from build123d import *

# Parameters (mm, degrees)
CROQUIS1_W                 = 48.280426218
CROQUIS1_H                 = 21.608022922
SALIENTE_EXTRUIR1_DEPTH    = 5
CROQUIS2_R                 = 2.974152903
CORTAR_EXTRUIR1_DEPTH      = 15
CORTAR_EXTRUIR1_DEPTH_BACK = 23
CROQUIS3_R                 = 3.556
CORTAR_EXTRUIR2_DEPTH      = 31.496
CORTAR_EXTRUIR2_DEPTH_BACK = 20.828
CROQUIS4_R                 = 3.556
CORTAR_EXTRUIR3_DEPTH      = 8.636
CORTAR_EXTRUIR3_DEPTH_BACK = 20.828
CROQUIS5_R                 = 4.117290135
SALIENTE_EXTRUIR2_DEPTH    = 8.636


with BuildPart() as part:
    # Croquis1 → Saliente-Extruir1 (new body)
    with BuildSketch(Plane(origin=(0, 0, 0), x_dir=(1, 0, 0), z_dir=(0, 1, 0))):
        Rectangle(CROQUIS1_W, CROQUIS1_H)
    extrude(amount=SALIENTE_EXTRUIR1_DEPTH)

    # Croquis2 → Cortar-Extruir1 (cut, two sides)
    with BuildSketch(Plane(origin=(0, 0, 0), x_dir=(1, 0, 0), z_dir=(0, 1, 0))) as cortar_extruir1_sk:
        with Locations((18.312839715, 0)):
            Circle(CROQUIS2_R)
        with Locations((-18.312839715, 0)):
            Circle(CROQUIS2_R)
    extrude(amount=CORTAR_EXTRUIR1_DEPTH, mode=Mode.SUBTRACT)
    extrude(cortar_extruir1_sk.sketch, amount=-CORTAR_EXTRUIR1_DEPTH_BACK, mode=Mode.SUBTRACT)

    # Croquis3 → Cortar-Extruir2 (cut, two sides)
    with BuildSketch(Plane(origin=(0, 0, 0), x_dir=(1, 0, 0), z_dir=(0, 1, 0))) as cortar_extruir2_sk:
        with Locations((18.312839715, 0)):
            Circle(CROQUIS3_R)
    extrude(amount=CORTAR_EXTRUIR2_DEPTH, mode=Mode.SUBTRACT)
    extrude(cortar_extruir2_sk.sketch, amount=-CORTAR_EXTRUIR2_DEPTH_BACK, mode=Mode.SUBTRACT)

    # Croquis4 → Cortar-Extruir3 (cut, two sides)
    with BuildSketch(Plane(origin=(0, 5, 0), x_dir=(1, 0, 0), z_dir=(0, 1, 0))) as cortar_extruir3_sk:
        with Locations((-18.312839715, 0)):
            Circle(CROQUIS4_R)
    extrude(amount=CORTAR_EXTRUIR3_DEPTH, mode=Mode.SUBTRACT)
    extrude(cortar_extruir3_sk.sketch, amount=-CORTAR_EXTRUIR3_DEPTH_BACK, mode=Mode.SUBTRACT)

    # Croquis5 → Saliente-Extruir2 (add)
    with BuildSketch(Plane.XY):
        Polygon((7.112251642, 9.190063188), (3.556125821, 15.349453788), (-3.556125821, 15.349453788), (-7.112251642, 9.190063188), (-3.556125821, 3.030672588), (3.556125821, 3.030672588), align=None)
        with Locations((0, 9.190063188)):
            Circle(CROQUIS5_R, mode=Mode.SUBTRACT)
    extrude(amount=SALIENTE_EXTRUIR2_DEPTH)


solid = part.part
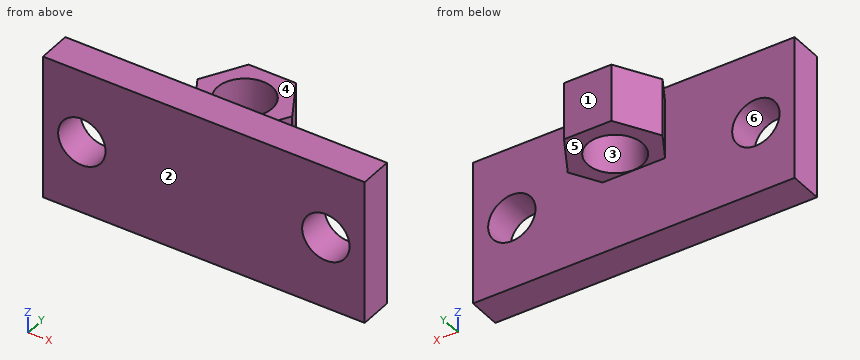
Model file for the job. Use its own axes, mm. Face numbers are marked on the shaded views. A direction names the side the tool comes from. Give positions to 0.01 mm unless a question says otherwise; leave off trailing zeros. Order: outer loops, then holes, each group sorted by start corner. A loop starts at its lowest first (then second) coordinate and runs counter-clockwise, first axis right, second up. Notation, with made-up numbers: (6, 54) - (41, 54) arc R10 cw to (41, 62) - close; hole circle Ø4 at (36.5, 12). An arc over 180 degrees is marked (long way). Return JSON: item names as keys, results as strings.
1) Flat gauge pins, fed straight in: P1, Ø8, axis at x = -0.5, y = 10, coming from the +Z side; P2, Ø3, axis at x = 1.5, z = 0.5, coming from the -Y side; P3, Ø11.5, axis at x = 18.31, z = 0, coming from the +Y side; P4, Ø5, axis at x = 9.5, y = 8, coming from the +Z side. Where does each tip first touch, or does it go through?
Geometry says:
{"P1": "z = 8.64", "P2": "y = 0", "P3": "y = 5", "P4": "through"}
2) Cut at B-B, the plane z = 3. Give the cut face in (x, y), plus the area to 3 significant figures.
Geometry says:
{"outline": "(-24.14, 0) - (-20.22, 0) - (-20.22, 5) - (-24.14, 5) - close; (-16.4, 0) - (16.4, 0) - (16.4, 5) - (4.69, 5) - (7.11, 9.19) - (3.56, 15.35) - (-3.56, 15.35) - (-7.11, 9.19) - (-4.69, 5) - (-16.4, 5) - close; (20.22, 0) - (24.14, 0) - (24.14, 5) - (20.22, 5) - close; hole circle Ø8.23 at (0, 9.19)", "area": "265 mm²"}
3) Cut at A-A, the plane x = 0. Give the cut face in (y, z), plus the area to 3 significant figures.
Geometry says:
{"outline": "(0, -10.8) - (5, -10.8) - (5, 0) - (5.07, 0) - (5.07, 8.64) - (5, 8.64) - (5, 10.8) - (0, 10.8) - close; (13.31, 0) - (15.35, 0) - (15.35, 8.64) - (13.31, 8.64) - close", "area": "126 mm²"}
4) Probe line 1 (X direction, y = 3.75, z = 0); line 2 (Y direction, x = 12, z = 0.75); line 3 (Y direction, x = 0, z = 3.5). List the from-to ranges inside material, lowest first. Write a range as from..to.
Geometry says:
{"line 1": "-24.14..-21.87, -14.76..14.76, 21.87..24.14", "line 2": "0..5", "line 3": "0..5.07, 13.31..15.35"}
5) Cut at C-C, the plane y = 2. Give the cut face in (x, z).
Geometry says:
{"outline": "(-24.14, -10.8) - (24.14, -10.8) - (24.14, 10.8) - (-24.14, 10.8) - close; hole circle Ø7.11 at (-18.31, 0); hole circle Ø7.11 at (18.31, 0)"}
6) 3-axis set-ups, long thin cutter, end or side, ignore diameter. For the marked faces 5 and 6: which of +Z, -Z, +X, -X, +Y, -Y reach the whole face in a straight line?
Geometry says:
{"face 5": "-Z, +X, -X, +Y", "face 6": "+Y, -Y"}
7) Cut at D-D, the plane z = -0.5. Give the cut face in (x, y).
Geometry says:
{"outline": "(-24.14, 0) - (-21.83, 0) - (-21.83, 5) - (-24.14, 5) - close; (-14.79, 0) - (14.79, 0) - (14.79, 5) - (-14.79, 5) - close; (21.83, 0) - (24.14, 0) - (24.14, 5) - (21.83, 5) - close"}
8) Pull direction Y, two halves, no side cores. Call the marked faces 1, 2, 3 and 4: pulls with the +Y half, pulls with the -Y half, needs draft (parallel to the pull), parting line crosses it, or undercut.
Geometry says:
{"face 1": "pulls with the +Y half", "face 2": "pulls with the -Y half", "face 3": "undercut", "face 4": "needs draft"}
